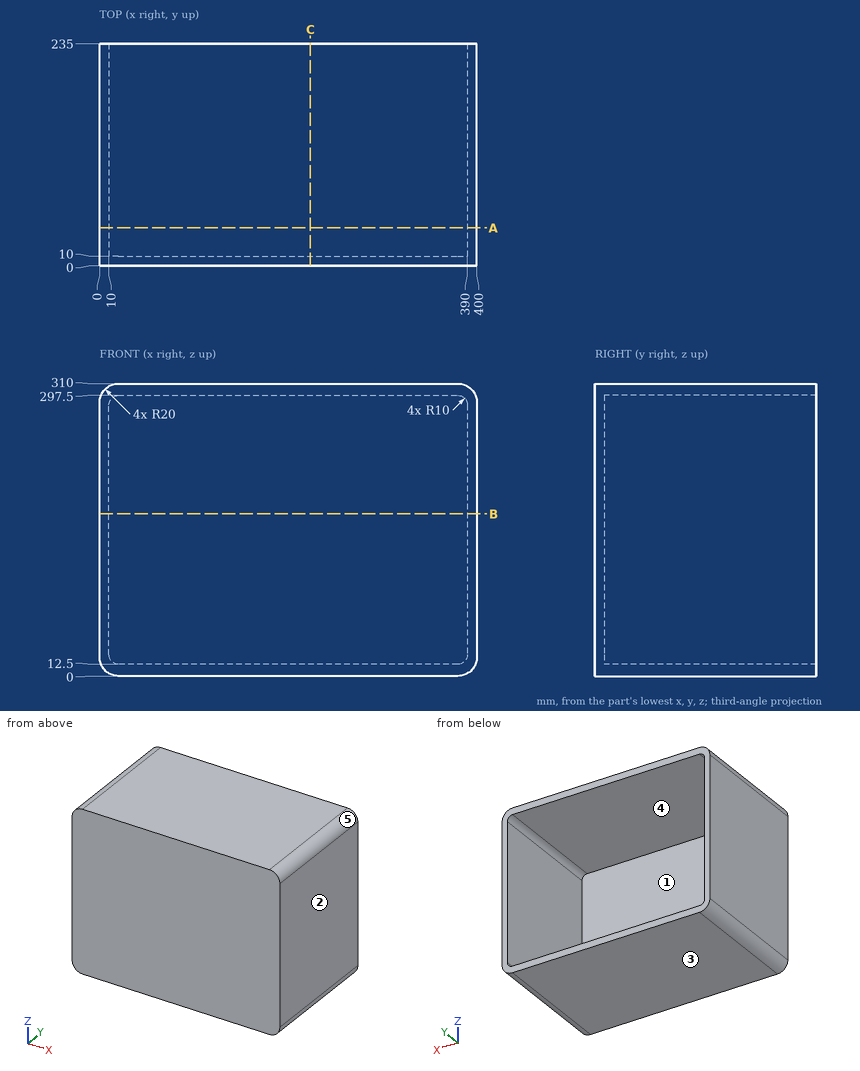
Here's the drawing with two shaded views (mm, measured from the low corner). I have some questions. A direction names the side the tool comes from. Coordinates: 2 decimals unless noted, no trailing zeros. Order: outer loops, then holes, each group sorted by start corner. A loop starts at its lowest first (then second) coordinate and runs counter-clockwise, first axis right, second up. Notation, with made-up numbers: (-34, -35.75) - (3, -35.75) arc R13 ccw to (3, -16.75) - close; hole circle Ø6 at (47, 29). An arc over 180 degrees is marked (long way). Answer in a Markdown table with one row per item.
1. If I drill on line 1 along Z through (x, y) = (213, 121); line 2 along X through (y, z) = (126.5, 161.5); line 3 along Y through (x, z) = (224, 217.5), over which ranges is the centre line in solid material (lowest first)?
Reply:
| item | result |
|---|---|
| line 1 | z = 0 to 12.5, 297.5 to 310 |
| line 2 | x = 0 to 10, 390 to 400 |
| line 3 | y = 0 to 10 |
2. Suppose I cut it at C-C (x = 223.5). Please give me the cut outline in (y, z), and give its area (4 significant figures).
Reply:
| item | result |
|---|---|
| outline | (0, 0) - (235, 0) - (235, 12.5) - (10, 12.5) - (10, 297.5) - (235, 297.5) - (235, 310) - (0, 310) - close |
| area | 8,725 mm^2 |
3. Suppose I cut it at A-A (y = 40). Please give me the cut outline in (x, z), and give its area (3 significant figures).
Reply:
| item | result |
|---|---|
| outline | (0, 20) arc R20 ccw to (20, 0) - (380, 0) arc R20 ccw to (400, 20) - (400, 290) arc R20 ccw to (380, 310) - (20, 310) arc R20 ccw to (0, 290) - close; hole (10, 22.5) arc R10 ccw to (20, 12.5) - (380, 12.5) arc R10 ccw to (390, 22.5) - (390, 287.5) arc R10 ccw to (380, 297.5) - (20, 297.5) arc R10 ccw to (10, 287.5) - close |
| area | 15,400 mm^2 |
4. Suppose I cut it at B-B (z = 172). Please give me the cut outline in (x, y).
Reply:
| item | result |
|---|---|
| outline | (0, 0) - (400, 0) - (400, 235) - (390, 235) - (390, 10) - (10, 10) - (10, 235) - (0, 235) - close |
5. For pin 1 (1 mm diameter, centred on x = 335.5, z = 66, fed in from +Y), with a flat end and sliding along its axis, tell me the tip position at first contact or that it passes through.
Reply:
| item | result |
|---|---|
| pin 1 | stops at y = 10 |
6. For the marked faces 1 and 2, which set-ups out of +Z, -Z, +X, -X, +Y, -Y let a thin tool reach every point of the face, with its end or its side?
Reply:
| item | result |
|---|---|
| face 1 | +Y |
| face 2 | +Z, -Z, +X, +Y, -Y |
7. If we mould it in two halves opening along Z, with no side actions, what happens to the marked faces 3, 4 and 5? For each: pulls with the +Z half, pulls with the -Z half, needs draft (parallel to the pull), parting line crosses it, or undercut.
Reply:
| item | result |
|---|---|
| face 3 | pulls with the -Z half |
| face 4 | undercut |
| face 5 | pulls with the +Z half |
